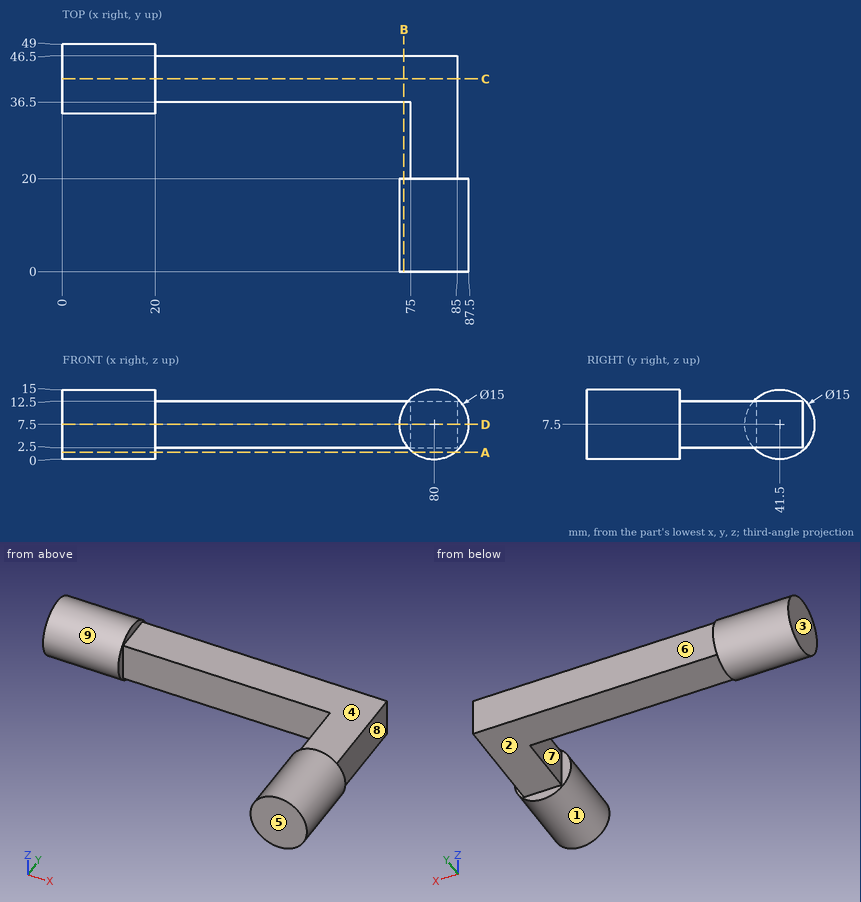
Here's the drawing with two shaded views (mm, measured from the low corner). I have some questions. A direction names the side the tool comes from. Give positions to 0.01 mm unless a question says otherwise; leave off trailing zeros. Order: outer loops, then holes, each group sorted by start corner. A loop starts at its lowest first (then second) coordinate and runs counter-clockwise, first axis right, second up. Notation, with made-up numbers: (-24, 17) -> (10, 17) arc R26 cw to (10, 48) -> close; hole circle Ø9 at (42.5, 49.5). An arc over 180 degrees is marked (long way). Use a Markdown table: item, result. Add a question column.
Item 1: If we mould it in two halves opening along Y, with no side actions, what happens to the marked faces 6, 7, 8 and 9? For each: pulls with the +Y half, pulls with the -Y half, needs draft (parallel to the pull), parting line crosses it, or undercut.
Item 2: Will these pins go through, and if not, where does the flat tip stop? pin 1 (3 mm diameter, centred on y = 23, z = 12.5, fed in from -X); pin 2 (5 mm diameter, centred on x = 46.5, z = 10, fed in from -Y); pin 3 (12 mm diameter, centred on x = 29.5, y = 39, fed in from +Z).
Item 3: Imagine slicing it at D-D on z = 7.5. Please give me the cut outline in (x, y).
Item 4: Imagine slicing it at C-C on y = 41.5. Please give me the cut outline in (x, z).
Item 5: I need wall thicknesses on line 1 (Y direction, x = 50, z = 11.75); line 2 (Z direction, x = 82, y = 45.5); line 3 (X direction, y = 25, z = 4.25). Which ranges of each line are inside material? Lowest first, please.
Item 6: Imagine slicing it at B-B on x = 73.5. Please give me the cut outline in (y, z).
Item 7: For the marked faces 1, 2, 3, 4 and 5, which set-ups out of +Z, -Z, +X, -X, +Y, -Y let a thin tool reach every point of the face, with its end or its side?
Item 8: Imagine slicing it at A-A on z = 1.5. Please give me the cut outline in (x, y), plus the area to 3 significant figures.
Data:
| question | item | result |
|---|---|---|
| 1 | face 6 | pulls with the +Y half |
| 1 | face 7 | undercut |
| 1 | face 8 | needs draft |
| 1 | face 9 | parting line crosses it |
| 2 | pin 1 | stops at x = 75 |
| 2 | pin 2 | stops at y = 36.5 |
| 2 | pin 3 | stops at z = 12.5 |
| 3 | outline | (0, 34) -> (20, 34) -> (20, 36.5) -> (75, 36.5) -> (75, 20) -> (72.5, 20) -> (72.5, 0) -> (87.5, 0) -> (87.5, 20) -> (85, 20) -> (85, 46.5) -> (20, 46.5) -> (20, 49) -> (0, 49) -> close |
| 4 | outline | (0, 0) -> (20, 0) -> (20, 2.5) -> (85, 2.5) -> (85, 12.5) -> (20, 12.5) -> (20, 15) -> (0, 15) -> close |
| 5 | line 1 | y = 36.5 to 46.5 |
| 5 | line 2 | z = 2.5 to 12.5 |
| 5 | line 3 | x = 75 to 85 |
| 6 | outline | (0, 3.76) -> (20, 3.76) -> (20, 11.24) -> (0, 11.24) -> close; (36.5, 2.5) -> (46.5, 2.5) -> (46.5, 12.5) -> (36.5, 12.5) -> close |
| 7 | face 1 | -Y |
| 7 | face 2 | -Z, +X, +Y |
| 7 | face 3 | +Z, -Z, -X, +Y, -Y |
| 7 | face 4 | +Z, +X, +Y |
| 7 | face 5 | +Z, -Z, +X, -X, -Y |
| 8 | outline | (0, 37) -> (20, 37) -> (20, 46) -> (0, 46) -> close; (75.5, 0) -> (84.5, 0) -> (84.5, 20) -> (75.5, 20) -> close |
| 8 | area | 360 mm² |
